```python
from build123d import *

# Parameters (mm, degrees)
F0_R      = 95
F1_DEPTH  = 355
F3_DEPTH  = 70
F4_R      = 85
F4_R_2    = 20
F5_DEPTH  = 40
F6_R      = 10
F7_DEPTH  = 25
F10_DEPTH = 98
F11_R     = 100
F11_R_2   = 95
F12_DEPTH = 70
F8_R      = 7.5
F13_DEPTH = 500
F14_R     = 5
F16_DEPTH = 47
F18_DEPTH = 75
F19_W     = 100
F19_H     = 50
F20_DEPTH = 22


# Not quite as in the source:
# - a feature names something its author has since deleted; it is built from what else it names


with BuildPart() as f1:
    # F0 (on Front) → F1 (new body)
    with BuildSketch(Plane.XZ):
        Circle(F0_R)
    extrude(amount=F1_DEPTH)

    # F2 (on face) → F3 (join)
    with BuildSketch(Plane.XZ.offset(355)):
        with BuildLine():
            Line((80, 51.2347538298), (80, 95))
            Line((80, 95), (46.4354390525, 95))
            Line((46.4354390525, 95), (0, 95))
            ThreePointArc((0, 95), (45.594398703, 83.3435708793), (80, 51.2347538298))
        make_face()
        with BuildLine():
            ThreePointArc((95, 0), (91.1729126441, 26.6926956301), (80, 51.2347538298))
            Line((80, 51.2347538298), (80, 50))
            Line((80, 50), (-80, 50))
            Line((-80, 50), (-80, 51.2347538298))
            ThreePointArc((-80, 51.2347538298), (-26.6926956301, -91.1729126441), (95, 0))
        make_face()
        with BuildLine():
            Line((80, 50), (80, 51.2347538298))
            ThreePointArc((80, 51.2347538298), (45.594398703, 83.3435708793), (0, 95))
            ThreePointArc((0, 95), (-45.594398703, 83.3435708793), (-80, 51.2347538298))
            Line((-80, 51.2347538298), (-80, 50))
            Line((-80, 50), (80, 50))
        make_face()
        with BuildLine():
            ThreePointArc((-80, 51.2347538298), (-45.594398703, 83.3435708793), (0, 95))
            Line((0, 95), (-46.4354390525, 95))
            Line((-46.4354390525, 95), (-80, 95))
            Line((-80, 95), (-80, 51.2347538298))
        make_face()
    extrude(amount=-F3_DEPTH)

    # F4 (on face) → F5 (cut)
    with BuildSketch(Plane.XZ.offset(355)):
        Circle(F4_R)
        Circle(F4_R_2, mode=Mode.SUBTRACT)
    extrude(amount=-F5_DEPTH, mode=Mode.SUBTRACT)

    # F6 (on face) → F7 (cut)
    with BuildSketch(Plane.XZ.offset(355)):
        Circle(F6_R)
    extrude(amount=-F7_DEPTH, mode=Mode.SUBTRACT)

    # F9 (on face) → F10 (join)
    with BuildSketch(Plane(origin=(0, 0, 0), x_dir=(-1, 0, 0), z_dir=(0, 1, 0))):
        with BuildLine():
            ThreePointArc((-80, 51.2347538298), (-45.594398703, 83.3435708793), (0, 95))
            Line((0, 95), (-75, 95))
            ThreePointArc((-75, 95), (-78.5355339059, 93.5355339059), (-80, 90))
            Line((-80, 90), (-80, 51.2347538298))
        make_face()
        with BuildLine():
            ThreePointArc((0, 95), (45.594398703, 83.3435708793), (80, 51.2347538298))
            Line((80, 51.2347538298), (80, 90))
            ThreePointArc((80, 90), (78.5355339059, 93.5355339059), (75, 95))
            Line((75, 95), (0, 95))
        make_face()
    extrude(amount=-F10_DEPTH)

    # F11 (on face) → F12 (join)
    with BuildSketch(Plane(origin=(0, -285, 0), x_dir=(-1, 0, 0), z_dir=(0, 1, 0))):
        Circle(F11_R)
        Circle(F11_R_2, mode=Mode.SUBTRACT)
    extrude(amount=-F12_DEPTH)

    # F8 (on face) → F13 (cut)
    with BuildSketch(Plane.XZ.offset(355)):
        with Locations((-62, 77)):
            Circle(F8_R)
        with Locations((62, 77)):
            Circle(F8_R)
    extrude(amount=-F13_DEPTH, mode=Mode.SUBTRACT)

    # F14
    f14_edges = [f1.edges().sort_by_distance(p)[0] for p in [
        (-80, -320, 95),
        (80, -320, 95),
    ]]
    fillet(f14_edges, radius=F14_R)

    # F15 (on face) → F16 (cut)
    with BuildSketch(Plane.XZ.offset(355)):
        with BuildLine():
            ThreePointArc((-80, 60), (0, 100), (80, 60))
            Line((80, 60), (80, 108.7283083646))
            Line((80, 108.7283083646), (-80, 108.7283083646))
            Line((-80, 108.7283083646), (-80, 60))
        make_face()
    extrude(amount=-F16_DEPTH, mode=Mode.SUBTRACT)

    # F17 (on face) → F18 (cut)
    with BuildSketch(Plane(origin=(0, 0, 0), x_dir=(-1, 0, 0), z_dir=(0, 1, 0))):
        with BuildLine():
            ThreePointArc((-80, 51.2347538298), (0, 95), (80, 51.2347538298))
            Line((80, 51.2347538298), (80, 103.6055907607))
            Line((80, 103.6055907607), (-80, 103.6055907607))
            Line((-80, 103.6055907607), (-80, 51.2347538298))
        make_face()
    extrude(amount=-F18_DEPTH, mode=Mode.SUBTRACT)

    # F19 (on face) → F20 (join)
    with BuildSketch(Plane.XY.offset(95)):
        with Locations((0, -123)):
            Rectangle(F19_W, F19_H)
    extrude(amount=-F20_DEPTH)


solid = f1.part
```
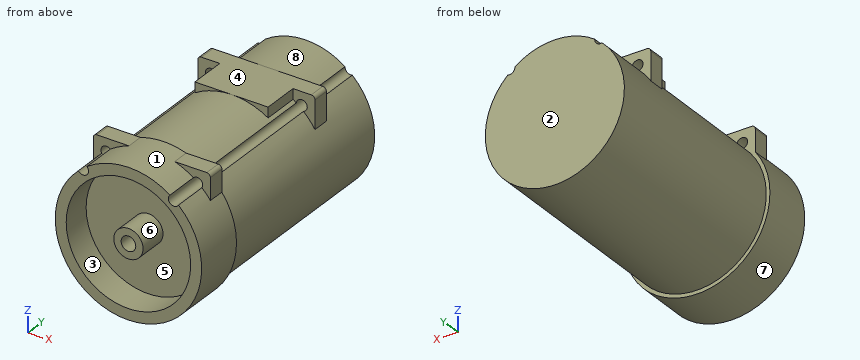
Geometry check sheet. Reference: the model listing, model coordinates, mm. Face numbers are marked on the shaded views. A direction names the side the tool comes from. Give positions to 0.01 mm unless a question says otherwise; leave off trailing zeros. Order: outer loops, then holes, each group sorted by start corner. A loop starts at its lowest first (then second) coordinate and runs counter-clockwise, first axis right, second up.
1. Section check B-B, the plane y = -203. Enter the section's corners in (x, z).
2. Section check A-A, the plane z = 0. Enter the section's corners in (x, y).
3. Access from +Z, -Z, +X, -X, +Y, -Y to the whole of each face (thin tool, end or side, straight path). Record for the marked faces 1, 2, 3 and 4.
4. Gauge pin test, flat ends, axial feed: pin 1 Ø7 at (y, z) = (-83, 70.5) entering from -X; pin 2 Ø7 at (y, z) = (-84, 72.5) entering from +X; pin 3 Ø10 at (x, y) = (-44, -112) entering from +Z; pin 4 Ø12 at (x, z) = (62, 77) entering from +Y. Record the tip position at first contact, or that the pin passes through.
5. Release check for a two-part mould opening along Z. For the marked faces 5, 6, 7 and 8 record: pulls with the +Z half, pulls with the -Z half, needs draft (parallel to the pull), parting line crosses it, or undercut.
6. Section check C-C, the plane z = -39. Enter the section's corners in (x, y).
7. Thickness scan on L1, parallel to Z at x = -1, y = -338 (3 decimals); L2, parallel to Y at x = 28.5, z = -45; L3, parallel to X at y = -198.5, z = 2.5. Record the ranges inside material, lowest first.
Values follow:
1. outline: (-64.36, 69.88) arc R95 ccw (long way) to (64.36, 69.88) arc R7.5 cw to (54.54, 77.78) arc R95 ccw to (-54.54, 77.78) arc R7.5 cw to start
2. outline: (-100, -355) - (-85, -355) - (-85, -315) - (-20, -315) - (-20, -355) - (-10, -355) - (-10, -330) - (10, -330) - (10, -355) - (20, -355) - (20, -315) - (85, -315) - (85, -355) - (100, -355) - (100, -285) - (95, -285) - (95, 0) - (-95, 0) - (-95, -285) - (-100, -285) - close
3. face 1: +Z, -Y
3. face 2: +Z, -Z, +X, -X, +Y
3. face 3: -Y
3. face 4: +Z, +X, -X, +Y
4. pin 1: stops at x = -80
4. pin 2: stops at x = 80
4. pin 3: stops at z = 95
4. pin 4: passes through
5. face 5: undercut
5. face 6: undercut
5. face 7: parting line crosses it
5. face 8: pulls with the +Z half
6. outline: (-92.08, -355) - (-75.52, -355) - (-75.52, -315) - (75.52, -315) - (75.52, -355) - (92.08, -355) - (92.08, -285) - (86.63, -285) - (86.63, 0) - (-86.63, 0) - (-86.63, -285) - (-92.08, -285) - close
7. L1: z = -99.995 to -84.994, -19.975 to -9.95, 9.95 to 19.975, 84.994 to 99.995
7. L2: y = -315 to 0
7. L3: x = -94.97 to 94.97
